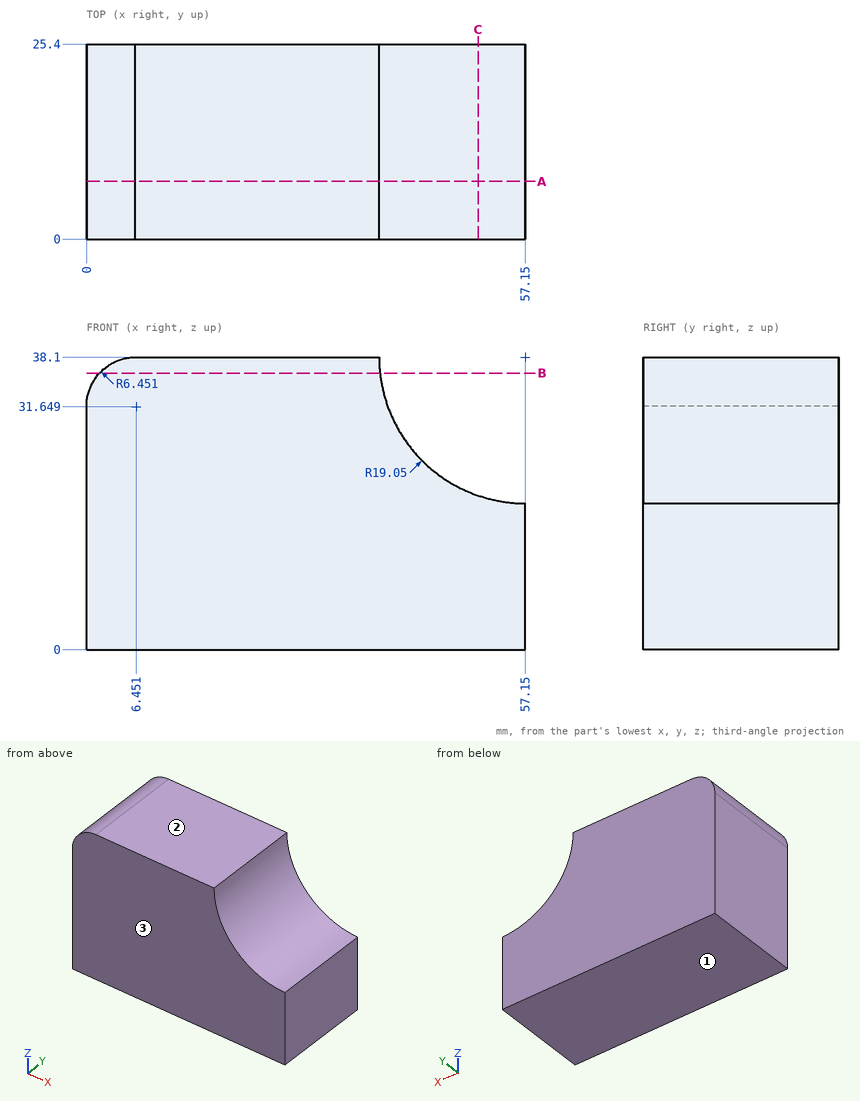
Here's the drawing with two shaded views (mm, measured from the low corner). I have some questions. Coordinates: 2 decimals unless noted, no trailing zeros. Loops run counter-clockwise (first coordinate to the right, second up) from the corner with the lowest first, then second, coordinate; pieces in that order, holes last. Notation, with made-up numbers: (50, 21.5) -> (101, 21.5) arc R23 cw to (101, 60.5) -> close; hole circle Ø2 at (72, 54). An arc over 180 degrees is marked (long way). Use one line per item in the form item = value. Start each with the question number.
(1) We'd pull the mould along Z, two halves only. Please class the marked faces 1, 2 and 3: pulls with the +Z half, pulls with the -Z half, needs draft (parallel to the pull), parting line crosses it, or undercut.
(2) Please list where these lines run through material, in increasing order: line 1 along Z through (x, y) = (41, 3.75) (1 decimal); line 2 along X through (y, z) = (14.25, 37.5) (1 decimal); line 3 along Z through (x, y) = (41.5, 10) (1 decimal).
(3) If we section it at A-A (y = 7.5): Please give me the cut outline in (x, z), then the cut area to 3 significant figures.
(4) If we section it at B-B (z = 36): Please give me the cut outline in (x, y).
(5) If we section it at C-C (x = 51): Please give me the cut outline in (y, z).
Verdict:
q1.face_1 = pulls with the -Z half
q1.face_2 = pulls with the +Z half
q1.face_3 = needs draft
q2.line_1 = 0 to 28
q2.line_2 = 3.7 to 38.1
q2.line_3 = 0 to 27.2
q3.outline = (0, 0) -> (57.15, 0) -> (57.15, 19.05) arc R19.05 cw to (38.1, 38.1) -> (6.35, 38.1) arc R6.45 ccw to (0, 31.75) -> close
q3.area = 1,880 mm²
q4.outline = (1.69, 0) -> (38.22, 0) -> (38.22, 25.4) -> (1.69, 25.4) -> close
q5.outline = (0, 0) -> (25.4, 0) -> (25.4, 20.07) -> (0, 20.07) -> close
